Could you check a few things on this model? Use its own coordinates, in mm. Coordinates: 2 decimals unless noted, no trailing zeros. Write each loop counter-clockwise with the first axis right and the second up, starting at its lowest first coordinate (ties: lowest second). Pieces come first, ordered by that corner, then holes.
```python
from build123d import *

# Parameters (mm, degrees)
F0_W     = 55
F0_H     = 40
F0_R     = 1.75
F1_DEPTH = 10
F2_R     = 5
F3_R     = 1.5
F4_DEPTH = 25


with BuildPart() as f1:
    # F0 (on Front) → F1 (new body)
    with BuildSketch(Plane.XZ):
        Rectangle(F0_W, F0_H)
        with Locations((-7.2848021371, -14.4358355429)):
            Circle(F0_R, mode=Mode.SUBTRACT)
        with BuildLine():
            ThreePointArc((-13.2479269502, -1.1975721574), (-13.2479153857, -1.2012452699), (-13.2479115309, -1.2049183986))
            ThreePointArc((-13.2479115309, -1.2049183986), (-16.7479076761, -1.2085915273), (-13.2479269502, -1.1975721574))
        make_face(mode=Mode.SUBTRACT)
        with Locations((8.0300629221, -14.3715454379)):
            Circle(F0_R, mode=Mode.SUBTRACT)
        with Locations((15.6318185876, -1.0763381886)):
            Circle(F0_R, mode=Mode.SUBTRACT)
        with Locations((-7.3961558654, 12.0902888507)):
            Circle(F0_R, mode=Mode.SUBTRACT)
        with BuildLine():
            ThreePointArc((6.8169535283, 5.8593717064), (4.871273383, 1.2216814773), (0.1990548634, -0.6395589675))
            ThreePointArc((0.1990548634, -0.6395589675), (-4.2373663264, 10.4970619355), (6.8169535283, 5.8593717064))
        make_face(mode=Mode.SUBTRACT)
        with Locations((7.9187091938, 12.1545789557)):
            Circle(F0_R, mode=Mode.SUBTRACT)
    extrude(amount=F1_DEPTH)

    # F2
    f2_edges = [f1.edges().sort_by_distance(p)[0] for p in [
        (-27.5, -5, 20),
        (-27.5, -5, -20),
        (27.5, -5, -20),
        (27.5, -5, 20),
    ]]
    fillet(f2_edges, radius=F2_R)

    # F3 (on face) → F4 (cut)
    with BuildSketch(Plane.XZ.offset(10)):
        with Locations((-24, 9.3585)):
            Circle(F3_R)
        with Locations((-24, -9.3585)):
            Circle(F3_R)
        with Locations((24, 9.3585)):
            Circle(F3_R)
        with Locations((24, -9.3585)):
            Circle(F3_R)
    extrude(amount=-F4_DEPTH, mode=Mode.SUBTRACT)


solid = f1.part
```
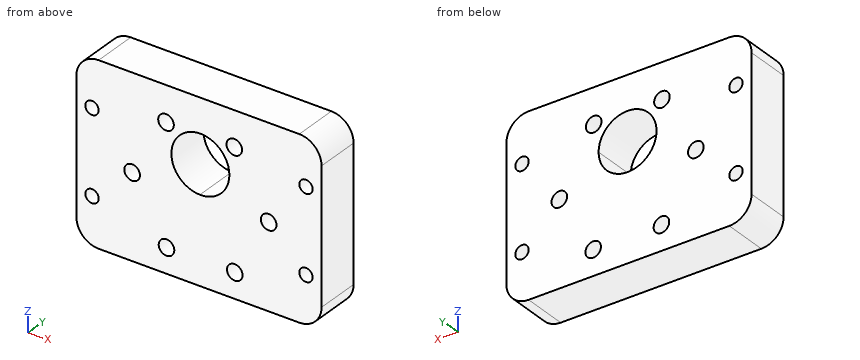
1. I want a section at D-D on y = -4. Give the number of separate pieces and of enclosed holes in the cut face, plus the area to 3 significant figures.
Verdict:
separate pieces: 1
enclosed holes: 11
area: 1,960 mm2
2. I want a section at B-B on x = 16. Please give me the cut outline in (y, z), plus the area to 3 significant figures.
Verdict:
outline: (-10, -20) - (0, -20) - (0, -2.79) - (-10, -2.79) - close; (-10, 0.63) - (0, 0.63) - (0, 20) - (-10, 20) - close
area: 366 mm2
3. Please list where these lines run through material, in increasing order: line 1 along X through (y, z) = (-5.5, -14.5); line 2 along Z through (x, y) = (-6.5, -7.25); line 3 along Z through (x, y) = (24, -3.5).
Verdict:
line 1: x = -27.5 to -9.03, -5.54 to 6.28, 9.78 to 27.5
line 2: z = -20 to -16, -12.87 to 10.59, 13.59 to 20
line 3: z = -19.77 to -10.86, -7.86 to 7.86, 10.86 to 19.77
4. For pin 1 (2 mm diameter, centred on x = 15.63, z = -1.08, fed in from +Y), with a flat end and sliding along its axis, tell me the tip position at first contact or that it passes through.
Verdict:
pin 1: passes through
5. I want a section at C-C on x = -24. Please give me the cut outline in (y, z), plus the area to 3 significant figures.
Verdict:
outline: (-10, -19.77) - (0, -19.77) - (0, -10.86) - (-10, -10.86) - close; (-10, -7.86) - (0, -7.86) - (0, 7.86) - (-10, 7.86) - close; (-10, 10.86) - (0, 10.86) - (0, 19.77) - (-10, 19.77) - close
area: 335 mm2
6. I want a section at A-A on z = 7. Please give me the cut outline in (x, y).
Verdict:
outline: (-27.5, -10) - (-6.08, -10) - (-6.08, 0) - (-27.5, 0) - close; (6.72, -10) - (27.5, -10) - (27.5, 0) - (6.72, 0) - close
